The figure shows three views and two pictorial views of one solid part (mm, origin at its lowest corner). Answer the questions. Give positions to 0.01 mm unless a question says otherwise; leave off trailing zeros. Write each loop counter-clockwise with the first axis right and the second up, starting at its lowest first coordinate (ties: lowest second). Pieces come first, ordered by that corner, then holes. Notation, with made-up numbers: (30.25, -21) -> (46.25, -21) arc R21 cw to (46.25, 17) -> close; hole circle Ø7 at (27, -13). An arc over 180 degrees is marked (long way). Write item = value, one per line. Start each with the question number.
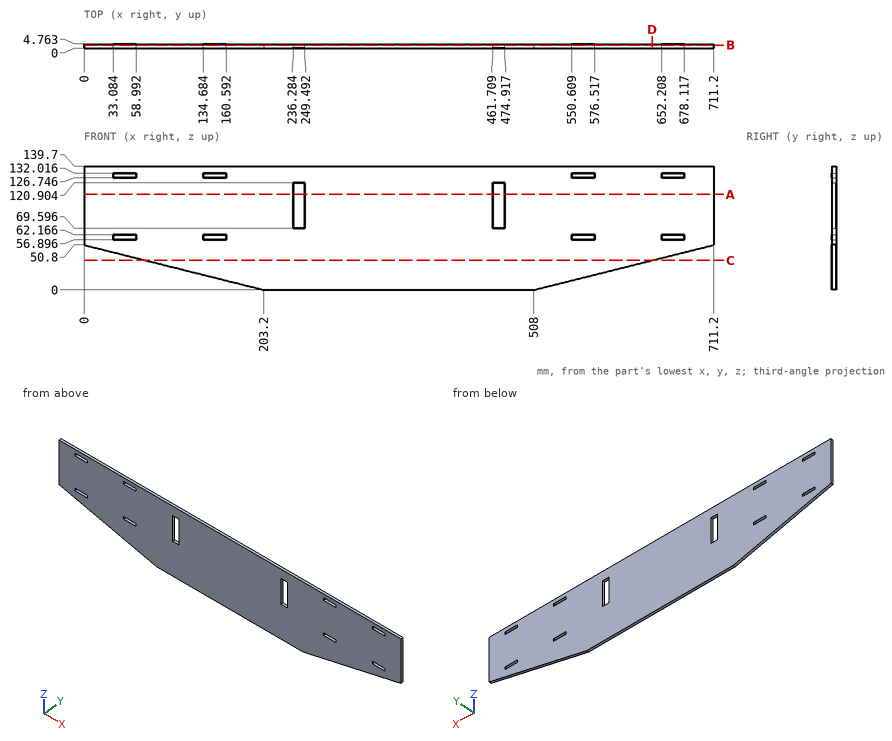
(1) Find the intervals of material crossed by line 1 along X through (y, z) = (1.8, 100); line 2 along X through (y, z) = (1.65, 128); line 3 along Z through (x, y) = (55.5, 4.5) (1 decimal), in increasing order.
(2) A cutting plane is placed at B-B, the plane y = 3.35. State how many separate pieces and enclosed holes the cut face has, then the cut area to 3 significant figures.
(3) A cutting plane is placed at C-C, the plane z = 33.5. Write down the section's boundary in (x, y).
(4) A cutting plane is placed at A-A, the plane z = 108. Write down the section's boundary in (x, y).
(5) A cutting plane is placed at D-D, the plane x = 641.5. Write down the section's boundary in (y, z) (1 decimal).
Results list:
q1.line_1 = 0 to 236.28, 249.49 to 461.71, 474.92 to 711.2
q1.line_2 = 0 to 33.08, 58.99 to 134.68, 160.59 to 550.61, 576.52 to 652.21, 678.12 to 711.2
q1.line_3 = 36.9 to 56.9, 62.2 to 126.7, 132 to 139.7
q2.separate_pieces = 1
q2.enclosed_holes = 10
q2.area = 86,600 mm²
q3.outline = (69.2, 0) -> (642, 0) -> (642, 4.76) -> (69.2, 4.76) -> close
q4.outline = (0, 0) -> (236.28, 0) -> (236.28, 4.76) -> (0, 4.76) -> close; (249.49, 0) -> (461.71, 0) -> (461.71, 4.76) -> (249.49, 4.76) -> close; (474.92, 0) -> (711.2, 0) -> (711.2, 4.76) -> (474.92, 4.76) -> close
q5.outline = (0, 33.4) -> (4.8, 33.4) -> (4.8, 139.7) -> (0, 139.7) -> close
